Autodesk Inventor part; units mm, degrees
ref_plane "YZ Plane" through (0, 0, 0) normal (1, 0, 0) x (0, 1, 0)
ref_plane "XZ Plane" through (0, 0, 0) normal (0, 1, 0) x (-1, 0, 0)
ref_plane "XY Plane" through (0, 0, 0) normal (0, 0, 1) x (1, 0, 0)
sketch "Sketch1" plane through (0, 0, 0) normal (0, 1, 0) x (-1, 0, 0)
  circle A0 centre (0, 0) radius 25
  dimension "d0" = 50
sketch "Sketch2" plane through (0, 0, 0) normal (0, 0, 1) x (1, 0, 0)
  point P0 (0, 0)
extrude "Extrusion1" add sketch "Sketch1" along normal blind 5
sketch "Sketch3" plane through (0, 5, 0) normal (0, 1, 0) x (1, 0, 0)
  circle A0 centre (0, 0) radius 3
  dimension "d3" = 6
extrude "Extrusion2" cut sketch "Sketch3" against normal blind 5
sketch "Sketch4" plane through (0, 5, 0) normal (0, 1, 0) x (1, 0, 0)
  circle A0 centre (17.9718, 0) radius 3
  point P0 (0, 0)
  dimension "d6" = 6
extrude "Extrusion3" cut sketch "Sketch4" against normal blind 5
CAD build for the part. Positions are in the model's coordinates, mm. Coordinates: 2 decimals unless noted, no trailing zeros. Loops run counter-clockwise (first coordinate to the right, second up) from the corner with the lowest first, then second, coordinate; pieces in that order, holes last. Notation, with made-up numbers: (-4.75, 81.25) -> (51.25, 81.25) arc R18 cw to (51.25, 88.25) -> close; hole circle Ø5 at (67.25, -36). An arc over 180 degrees is marked (long way). One line per item, written item: value.
1. Slice it at B-B on z = 0. Write the cut outline in (x, y), and give its area (3 significant figures).
Answers:
outline: (-25, 0) -> (-3, 0) -> (-3, 5) -> (-25, 5) -> close; (3, 0) -> (14.97, 0) -> (14.97, 5) -> (3, 5) -> close; (20.97, 0) -> (25, 0) -> (25, 5) -> (20.97, 5) -> close
area: 190 mm^2
2. Drill centre lines: line 1 (Z direction, x = 0, y = 3.05); line 2 (X direction, y = 3.05, z = 0.5) (3 decimals); line 3 (X direction, y = 1.3, z = 2.5). Where is each one in solid material? Low to high. Write a range as [from, to].
Answers:
line 1: z = [-25, -3], [3, 25]
line 2: x = [-24.995, -2.958], [2.958, 15.014], [20.93, 24.995]
line 3: x = [-24.87, -1.66], [1.66, 16.31], [19.63, 24.87]
3. Pull direction Z, two halves, no side cores. Call faces 1 (the face through (-3, 3, 0)), 2 (the face through (-5, 0, 0)), 3 (the face through (-23.846, 2.465, -7.509)): pulls with the +Z half, pulls with the -Z half, needs draft (parallel to the pull), parting line crosses it, or undercut.
Answers:
face 1: undercut
face 2: needs draft
face 3: parting line crosses it
4. Slice it at C-C on y = 2.1. Write the cut outline in (x, z), and give its area (3 significant figures).
Answers:
outline: circle Ø50 at (0, 0); hole circle Ø6 at (0, 0); hole circle Ø6 at (17.97, 0)
area: 1,910 mm^2
5. Slice it at A-A on x = 0. Write the cut outline in (y, z), and give its area (3 significant figures).
Answers:
outline: (0, -25) -> (5, -25) -> (5, -3) -> (0, -3) -> close; (0, 3) -> (5, 3) -> (5, 25) -> (0, 25) -> close
area: 220 mm^2
6. Flat gauge pin, fed straight in: P1, Ø1, axis at y = 3, z = 11.5, coming from the -X side. Where does the tip first touch, or does it go through?
Answers:
P1: stops at x = -22.45
7. Slice it at D-D on x = 12. Write the cut outline in (y, z).
Answers:
outline: (0, -21.93) -> (5, -21.93) -> (5, 21.93) -> (0, 21.93) -> close
